Design review of the part built by this model. Coordinates are the model's own, in mm. Give positions to 0.01 mm unless a question says otherwise; leave off trailing zeros. Loops run counter-clockwise (first coordinate to the right, second up) from the corner with the lowest first, then second, coordinate; pieces in that order, holes last. Notation, with made-up numbers: (21.5, 88.5) -> (69.5, 88.5) arc R23 ccw to (69.5, 98.5) -> close; hole circle Ø4 at (-31, -22). An arc over 180 degrees is marked (long way). Use a Markdown table: item, result. Add a question column.
1. Add section B-B (x = 70). State the section outline as (y, z) points, and give its area (3 significant figures).
2. Add section C-C (z = 2.75). State the section outline as (x, y) points.
3. Add section D-D (y = 89). State the section outline as (x, z) points.
4. Add section A-A (y = 48). State the section outline as (x, z) points, and give its area (3 significant figures).
5. For pin 1 Ø4.5 at (x, y) = (89, 89) entering from +Z; pin 2 Ø3.5 at (x, y) = (89, 7) entering from -Z, all flat-tipped, find the tip position at first contact; note any pin that passes through.
6. Draft analysis for pull direction X (two halves, no side actions). For faces 1 (the cylindrical face through (87.925, 90.686, 3.944)), 2 (the flat face through (96, 47, 4)), 3 (the cylindrical face through (9, 7, 4)), 4 (the flat face through (26, 70, 0)), state which applies: pulls with the +X half, pulls with the -X half, needs draft (parallel to the pull), parting line crosses it, or undercut.
7. To check wall thickness, follow line 1 (Y direction, x = 7, z = 3); line 2 (X direction, y = 87.5, z = 7.25); line 3 (X direction, y = 64, z = 4.75). State the ranges of each line that lie inside material, in increasing order.
```python
from build123d import *

# Parameters (mm, degrees)
SKETCH1_W           = 96
SKETCH1_H           = 96
BOSS_EXTRUDE1_DEPTH = 0.6
CUT_EXTRUDE1_DEPTH  = 74.6
SKETCH3_R           = 27.3
CUT_EXTRUDE2_DEPTH  = 74.6
SKETCH4_R           = 2
CUT_EXTRUDE3_DEPTH  = 74.6
SKETCH5_R           = 37.3
SKETCH5_R_2         = 27.3
BOSS_EXTRUDE3_DEPTH = 2.5
BOSS_EXTRUDE3_DRAFT = 42
BOSS_EXTRUDE4_START = 7.4
SKETCH8_R           = 27.3
BOSS_EXTRUDE4_DEPTH = 7.4
SKETCH9_R           = 2
CUT_EXTRUDE4_DEPTH  = 137


with BuildPart() as part:
    # Sketch1 → Boss-Extrude1 (new body)
    with BuildSketch(Plane.XY):
        with Locations((48, 48)):
            Rectangle(SKETCH1_W, SKETCH1_H)
    extrude(amount=BOSS_EXTRUDE1_DEPTH)

    # Sketch2 → Cut-Extrude1 (cut)
    with BuildSketch(Plane.XY.offset(0.6)):
        with BuildLine():
            Line((10, 96), (0, 96))
            Line((0, 96), (0, 86))
            ThreePointArc((0, 86), (2.928932188, 93.071067812), (10, 96))
        make_face()
        with BuildLine():
            Line((86, 96), (96, 96))
            Line((96, 96), (96, 86))
            ThreePointArc((96, 86), (93.071067812, 93.071067812), (86, 96))
        make_face()
        with BuildLine():
            Line((86, 0), (96, 0))
            Line((96, 0), (96, 10))
            ThreePointArc((96, 10), (93.071067812, 2.928932188), (86, 0))
        make_face()
        with BuildLine():
            Line((0, 0), (10, 0))
            ThreePointArc((10, 0), (2.928932188, 2.928932188), (0, 10))
            Line((0, 10), (0, 0))
        make_face()
    extrude(amount=-CUT_EXTRUDE1_DEPTH, mode=Mode.SUBTRACT)

    # Sketch3 → Cut-Extrude2 (cut)
    with BuildSketch(Plane.XY.offset(0.6)):
        with Locations((48, 48)):
            Circle(SKETCH3_R)
    extrude(amount=-CUT_EXTRUDE2_DEPTH, mode=Mode.SUBTRACT)

    # Sketch4 → Cut-Extrude3 (cut)
    with BuildSketch(Plane(origin=(0, 0, 0), x_dir=(-1, 0, 0), z_dir=(0, 0, -1))):
        with Locations((-89, 89)):
            Circle(SKETCH4_R)
        with Locations((-7, 89)):
            Circle(SKETCH4_R)
        with Locations((-7, 7)):
            Circle(SKETCH4_R)
        with Locations((-89, 7)):
            Circle(SKETCH4_R)
    extrude(amount=-CUT_EXTRUDE3_DEPTH, mode=Mode.SUBTRACT)


with BuildPart() as boss_extrude3_tool:
    # Sketch5 → Boss-Extrude3 (with draft: the straight prism first)
    with BuildSketch(Plane.XY.offset(0.6)):
        with Locations((48, 48)):
            Circle(SKETCH5_R)
        with Locations((48, 48)):
            Circle(SKETCH5_R_2, mode=Mode.SUBTRACT)
    extrude(amount=BOSS_EXTRUDE3_DEPTH)
    # Boss-Extrude3: the draft: its side faces are tilted about the plane it starts from
    boss_extrude3_sides = [boss_extrude3_tool.faces().sort_by_distance(p)[0] for p in [
        (10.7, 48, 1.85),
        (20.7, 48, 1.85),
    ]]
    draft(boss_extrude3_sides, Plane.XY.offset(0.6), BOSS_EXTRUDE3_DRAFT)


with BuildPart() as part_1:
    add(part.part)

    # Boss-Extrude3: add boss_extrude3_tool
    add(boss_extrude3_tool.part)

    # Sketch8 → Boss-Extrude4 (add)
    with BuildSketch(Plane.XY.offset(0.6).offset(BOSS_EXTRUDE4_START)):
        with BuildLine():
            Line((0, 86), (0, 10))
            ThreePointArc((0, 10), (2.928932188, 2.928932188), (10, 0))
            Line((10, 0), (86, 0))
            ThreePointArc((86, 0), (93.071067812, 2.928932188), (96, 10))
            Line((96, 10), (96, 86))
            ThreePointArc((96, 86), (93.071067812, 93.071067812), (86, 96))
            Line((86, 96), (10, 96))
            ThreePointArc((10, 96), (2.928932188, 93.071067812), (0, 86))
        make_face()
        with Locations((48, 48)):
            Circle(SKETCH8_R, mode=Mode.SUBTRACT)
    extrude(amount=-BOSS_EXTRUDE4_DEPTH)

    # Sketch9 → Cut-Extrude4 (cut, through all)
    with BuildSketch(Plane(origin=(0, 0, 0), x_dir=(-1, 0, 0), z_dir=(0, 0, -1))):
        with Locations((-7, 89)):
            Circle(SKETCH9_R)
        with Locations((-89, 89)):
            Circle(SKETCH9_R)
        with Locations((-89, 7)):
            Circle(SKETCH9_R)
        with Locations((-7, 7)):
            Circle(SKETCH9_R)
    extrude(amount=-CUT_EXTRUDE4_DEPTH, mode=Mode.SUBTRACT)


solid = part_1.part
```
Taken from the geometry:
| question | item | result |
|---|---|---|
| 1 | outline | (0, 0) -> (31.84, 0) -> (31.84, 8) -> (0, 8) -> close; (64.16, 0) -> (96, 0) -> (96, 8) -> (64.16, 8) -> close |
| 1 | area | 509 mm^2 |
| 2 | outline | (0, 10) arc R10 ccw to (10, 0) -> (86, 0) arc R10 ccw to (96, 10) -> (96, 86) arc R10 ccw to (86, 96) -> (10, 96) arc R10 ccw to (0, 86) -> close; hole circle Ø4 at (7, 7); hole circle Ø4 at (7, 89); hole circle Ø54.6 at (48, 48); hole circle Ø4 at (89, 7); hole circle Ø4 at (89, 89) |
| 3 | outline | (0.46, 0) -> (5, 0) -> (5, 8) -> (0.46, 8) -> close; (9, 0) -> (87, 0) -> (87, 8) -> (9, 8) -> close; (91, 0) -> (95.54, 0) -> (95.54, 8) -> (91, 8) -> close |
| 4 | outline | (0, 0) -> (20.7, 0) -> (20.7, 8) -> (0, 8) -> close; (75.3, 0) -> (96, 0) -> (96, 8) -> (75.3, 8) -> close |
| 4 | area | 331 mm^2 |
| 5 | pin 1 | stops at z = 8 |
| 5 | pin 2 | passes through |
| 6 | face 1 | undercut |
| 6 | face 2 | pulls with the +X half |
| 6 | face 3 | undercut |
| 6 | face 4 | needs draft |
| 7 | line 1 | y = 0.46 to 5, 9 to 87, 91 to 95.54 |
| 7 | line 2 | x = 0.11 to 5.68, 8.32 to 87.68, 90.32 to 95.89 |
| 7 | line 3 | x = 0 to 25.88, 70.12 to 96 |
